Build history of the part. All positions in model axes, mm. Face numbers are marked on the shaded views. A direction names the side the tool comes from. Give positions to 0.01 mm unless a question says otherwise; leave off trailing zeros. Loops run counter-clockwise (first coordinate to the right, second up) from the corner with the lowest first, then second, coordinate; pieces in that order, holes last. Notation, with made-up numbers: (0.25, 35.25) -> (18.25, 35.25) arc R29 ccw to (18.25, 74.25) -> close; hole circle Ø6 at (44.5, 68). An arc over 180 degrees is marked (long way). Answer as a JSON object with one key per item and string values. Group by question number.
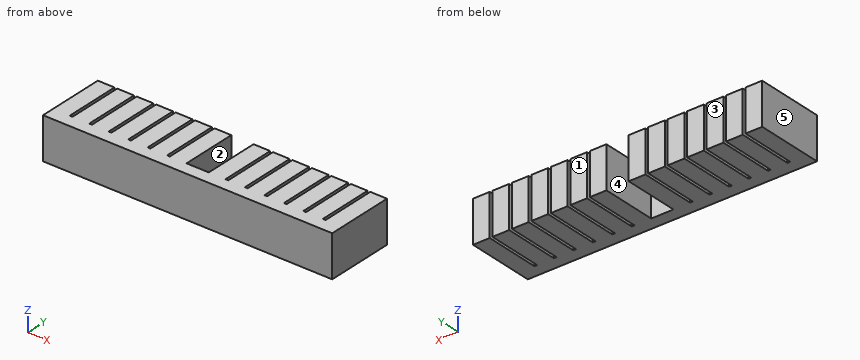
from build123d import *

# Parameters (mm, degrees)
BOSS_EXTRUDE1_DEPTH     = 7.5
LPATTERN1_COUNT         = 8
LPATTERN1_PITCH         = 7
LPATTERN1_COL_COUNT     = 8
LPATTERN1_COL_PITCH     = 7
SHELL2_T                = -1
CUT_EXTRUDE2_DEPTH      = 15
CUT_EXTRUDE2_DEPTH_BACK = 58.608593109
SKETCH3_W               = 0.5
SKETCH3_H               = 4.5
SKETCH4_W               = 13
SKETCH4_H               = 2.5
BOSS_EXTRUDE2_DEPTH     = 1
SKETCH5_W               = 13
SKETCH5_H               = 2.5
BOSS_EXTRUDE3_DEPTH     = 1
SKETCH8_W               = 6
SKETCH8_H               = 15
BOSS_EXTRUDE5_DEPTH     = 2
LPATTERN2_COUNT         = 15
LPATTERN2_PITCH         = 7
SKETCH10_W              = 6
SKETCH10_H              = 15
CUT_EXTRUDE4_DEPTH      = 20
SKETCH11_W              = 13
SKETCH11_H              = 1
BOSS_EXTRUDE6_DEPTH     = 4


# Read off the part's stored shape, not the designer's step: Split1
with BuildPart() as part:
    # Sketch1 → Boss-Extrude1 (new, symmetric)
    with BuildSketch(Plane.XY):
        Polygon((0, 0), (-3.5, 0), (-3.5, 4.5), (-3, 4.5), (-3, 22.5), (3, 22.5), (3, 4.5), (3.5, 4.5), (3.5, 0), align=None)
    boss_extrude1 = extrude(amount=BOSS_EXTRUDE1_DEPTH, both=True)

    # LPattern1: Boss-Extrude1 ×8
    with Locations(*[(-i * LPATTERN1_PITCH, 0, 0) for i in range(1, LPATTERN1_COUNT)]):
        add(boss_extrude1)


with BuildPart() as lpattern1_col_1:
    # LPattern1 col: pattern copy
    add(boss_extrude1.moved(Location(Vector(1, 0, 0) * (1 * LPATTERN1_COL_PITCH))))


with BuildPart() as lpattern1_col_2:
    # LPattern1 col: pattern copy
    add(boss_extrude1.moved(Location(Vector(1, 0, 0) * (2 * LPATTERN1_COL_PITCH))))


with BuildPart() as lpattern1_col_3:
    # LPattern1 col: pattern copy
    add(boss_extrude1.moved(Location(Vector(1, 0, 0) * (3 * LPATTERN1_COL_PITCH))))


with BuildPart() as lpattern1_col_4:
    # LPattern1 col: pattern copy
    add(boss_extrude1.moved(Location(Vector(1, 0, 0) * (4 * LPATTERN1_COL_PITCH))))


with BuildPart() as lpattern1_col_5:
    # LPattern1 col: pattern copy
    add(boss_extrude1.moved(Location(Vector(1, 0, 0) * (5 * LPATTERN1_COL_PITCH))))


with BuildPart() as lpattern1_col_6:
    # LPattern1 col: pattern copy
    add(boss_extrude1.moved(Location(Vector(1, 0, 0) * (6 * LPATTERN1_COL_PITCH))))


with BuildPart() as lpattern1_col_7:
    # LPattern1 col: pattern copy
    add(boss_extrude1.moved(Location(Vector(1, 0, 0) * (7 * LPATTERN1_COL_PITCH))))


with BuildPart() as part_1:
    add(part.part)

    # LPattern1 col united with what the copie: union LPattern1 col_1, LPattern1 col_2, LPattern1 col_3, LPattern1 col_4, LPattern1 col_5, LPattern1 col_6, LPattern1 col_7
    add(lpattern1_col_1.part)
    add(lpattern1_col_2.part)
    add(lpattern1_col_3.part)
    add(lpattern1_col_4.part)
    add(lpattern1_col_5.part)
    add(lpattern1_col_6.part)
    add(lpattern1_col_7.part)

    # Shell2
    shell2_openings = [part_1.faces().sort_by_distance(p)[0] for p in [
        (52.5, 2.25, 0),
        (-52.5, 2.25, 0),
    ]]
    offset(amount=SHELL2_T, openings=shell2_openings, kind=Kind.INTERSECTION)

    # Sketch3 → Cut-Extrude2 (cut, two sides: drawn at the far end of the back side and taken through both)
    with BuildSketch(Plane.XY.offset(-CUT_EXTRUDE2_DEPTH_BACK)):
        with Locations((-52.25, 2.25)):
            Rectangle(SKETCH3_W, SKETCH3_H)
        with Locations((52.25, 2.25)):
            Rectangle(SKETCH3_W, SKETCH3_H)
    extrude(amount=CUT_EXTRUDE2_DEPTH + CUT_EXTRUDE2_DEPTH_BACK, mode=Mode.SUBTRACT)

    # Sketch4 → Boss-Extrude2 (add)
    with BuildSketch(Plane.ZY.offset(52)):
        with Locations((0, 2.25)):
            Rectangle(SKETCH4_W, SKETCH4_H)
    extrude(amount=-BOSS_EXTRUDE2_DEPTH)

    # Sketch5 → Boss-Extrude3 (add)
    with BuildSketch(Plane(origin=(52, 0, 0), x_dir=(0, 0, -1), z_dir=(1, 0, 0))):
        with Locations((0, 2.25)):
            Rectangle(SKETCH5_W, SKETCH5_H)
    extrude(amount=-BOSS_EXTRUDE3_DEPTH)

    # Sketch8 → Boss-Extrude5 (add)
    with BuildSketch(Plane(origin=(0, 22.5, 0), x_dir=(1, 0, 0), z_dir=(0, 1, 0))):
        with Locations((-49, 0)):
            Rectangle(SKETCH8_W, SKETCH8_H)
    boss_extrude5 = extrude(amount=BOSS_EXTRUDE5_DEPTH)

    # LPattern2: Boss-Extrude5 ×15
    with Locations(*[(i * LPATTERN2_PITCH, 0, 0) for i in range(1, LPATTERN2_COUNT)]):
        add(boss_extrude5)


with BuildPart() as body_2:
    # Split1: the piece on the far side of the plane
    add(part_1.part)
    split(bisect_by=Plane(origin=(0, 1, 0), x_dir=(1, 0, 0), z_dir=(0, 1, 0)), keep=Keep.BOTTOM)


with BuildPart() as part_2:
    add(part_1.part)

    # Split1
    split(bisect_by=Plane(origin=(0, 1, 0), x_dir=(1, 0, 0), z_dir=(0, 1, 0)), keep=Keep.TOP)

    # Sketch10 → Cut-Extrude4 (cut)
    with BuildSketch(Plane(origin=(0, 24.5, 0), x_dir=(1, 0, 0), z_dir=(0, 1, 0))):
        Rectangle(SKETCH10_W, SKETCH10_H)
    extrude(amount=-CUT_EXTRUDE4_DEPTH, mode=Mode.SUBTRACT)

    # Sketch11 → Boss-Extrude6 (add)
    with BuildSketch(Plane(origin=(-2, 0, 0), x_dir=(0, 0, -1), z_dir=(1, 0, 0))):
        with Locations((0, 4)):
            Rectangle(SKETCH11_W, SKETCH11_H)
    extrude(amount=BOSS_EXTRUDE6_DEPTH)


with BuildPart() as body_2_1:
    add(body_2.part)

    # Combine1: union part
    add(part_2.part)


solid = body_2_1.part
(1) Saw through at C-C on y = 13.75. Give the number of separate pieces and of enclosed holes in the cut face, plus the area to 3 significant figures.
(2) Probe line 1 along Z through (x, y) = (43, 6.75); line 2 along Y through (x, z) = (39.5, -4.5); line 3 along Y through (x, z) = (20, -6). List the from-to ranges inside material, lowest first. Write a range as [from, to].
(3) Pull direction X, two halves, no side cores. Call the marked faces 3, 4 and 5: pulls with the +X half, pulls with the -X half, needs draft (parallel to the pull), parting line crosses it, or undercut.
(4) 3-axis set-ups, long thin cutter, end or side, ignore diameter. For the marked faces 1 and 2: which of +Z, -Z, +X, -X, +Y, -Y reach the whole face in a straight line?
(5) Pin check, flat tip, straight feed: pin 1 (0.8 mm diameter, centred on x = 10.5, z = 0, fed in from +Y). Stop position of the tip, or through.
(6) Saw through at A-A on x = -8. List the corners of the cut face in (y, z).
(7) Saw through at B-B on y = 2.5. List the corners of the cut face in (x, z).
Calculated:
{
 "1": {"separate pieces": "14", "enclosed holes": "14", "area": "532 mm^2"},
 "2": {"line 1": "z = [-7.5, -6.5], [6.5, 7.5]", "line 2": "y = [0, 1], [3.5, 24.5]", "line 3": "y = [0, 1], [21.5, 24.5]"},
 "3": {"face 3": "needs draft", "face 4": "undercut", "face 5": "pulls with the -X half"},
 "4": {"face 1": "+Z, -Z, +X, -X, +Y", "face 2": "+Z, -Z, +Y"},
 "5": {"pin 1": "stops at y = 4.5"},
 "6": {"outline": "(0, -7.5) -> (24.5, -7.5) -> (24.5, 7.5) -> (0, 7.5) -> close; hole (1, -6.5) -> (21.5, -6.5) -> (21.5, 6.5) -> (1, 6.5) -> close"},
 "7": {"outline": "(-52, -7.5) -> (52, -7.5) -> (52, 7.5) -> (-52, 7.5) -> close; hole (-51, -6.5) -> (51, -6.5) -> (51, 6.5) -> (-51, 6.5) -> close"}
}
